Source: three-view drawing plus pictorial views. Frame: mm from the lowest corner of the part. Give positions to 0.01 mm unless a question says otherwise; leave off trailing zeros. Order: outer loops, then holes, each group sorted by start corner. A loop starts at its lowest first (then second) coordinate and runs counter-clockwise, first axis right, second up. Notation, with made-up numbers: (28, -9.5) - (87, -9.5) arc R12 ccw to (87, -5.5) - close; hole circle Ø5 at (38.5, 62). An arc over 180 degrees is marked (long way). Use one line per item in the form item = value.
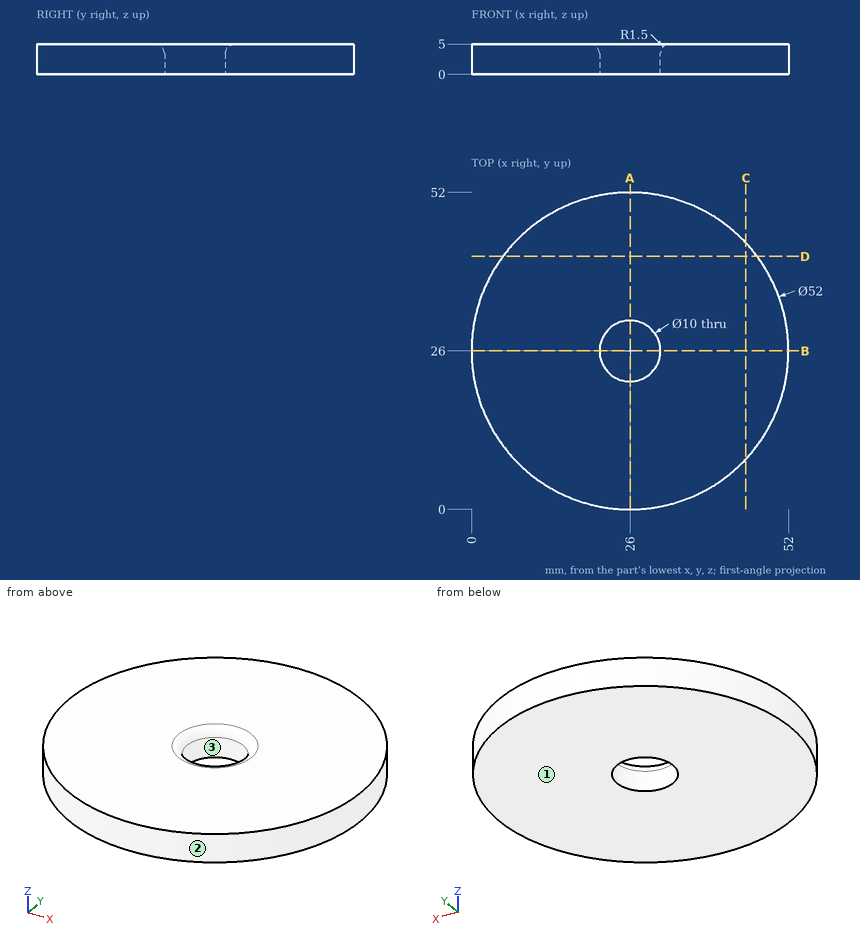
(1) Ray query, line 1 along Y through (x, z) = (26, 1.6); line 2 along Y through (x, z) = (29, 0.4); line 3 along X through (y, z) = (32, 1.1). Return the intervals inside material, ascending.
Computed values:
line_1 = 0 to 21, 31 to 52
line_2 = 0.17 to 22, 30 to 51.83
line_3 = 0.7 to 51.3
(2) Pull-direction query (Y, two-part tool) for the marked faces 1, 2 and 3; classes: released by +Y, released by -Y, zero draft, split by the parting line, or undercut.
Computed values:
face_1 = zero draft
face_2 = split by the parting line
face_3 = undercut
(3) Cut plane D-D on y = 41.5. Output: boundary loops of the cut face in (x, z).
Computed values:
outline = (5.13, 0) - (46.87, 0) - (46.87, 5) - (5.13, 5) - close
(4) Contact query for flat-ended pins moving along their axis: pin 1 Ø3 at (x, z) = (29.5, 1) entering from -Y; pin 2 Ø3 at (y, z) = (28, 2.5) entering from +X; pin 3 Ø2 at (y, z) = (35.5, 2.5) entering from +X. Output: stop coordinate, or through.
Computed values:
pin_1 = 0.08
pin_2 = 52
pin_3 = 50.57
(5) Cut plane A-A on x = 26. Output: boundary loops of the cut face in (y, z), plus the area to 3 significant figures.
Computed values:
outline = (0, 0) - (21, 0) - (21, 3.5) arc R1.5 ccw to (19.5, 5) - (0, 5) - close; (31, 0) - (52, 0) - (52, 5) - (32.5, 5) arc R1.5 ccw to (31, 3.5) - close
area = 209 mm²
(6) Cut plane C-C on x = 45. Output: boundary loops of the cut face in (y, z), plus the area to 3 significant figures.
Computed values:
outline = (8.25, 0) - (43.75, 0) - (43.75, 5) - (8.25, 5) - close
area = 177 mm²
